Study the drawing (mm; zero at the part's minimum x, y, z) and answer. Coordinates: 2 decimals unless noted, no trailing zeros. Order: outer loops, then holes, each group sorted by start corner. A loop starts at its lowest first (then second) coordinate and runs counter-clockwise, first axis right, second up.
1. Flat-ended cylindrical pins translate along their axes: pin 1 Ø4.5 at (x, z) = (4.5, 2.5) entering from +Y; pin 2 Ø2.5 at (x, z) = (14.5, 2.5) entering from +Y. Find the tip coordinate at first contact, or state that the pin passes through.
2. The part is cut by section D-D, the plane x = 13.5. Give the vertices of the cut face in (y, z), then the cut area to 3 significant figures.
3. The part is cut by section C-C, the plane z = 17.5. Give the vertices of the cut face in (x, y), then the cut area to 3 significant figures.
4. The part is cut by section B-B, the plane x = 9.5. Give the vertices of the cut face in (y, z), then the cut area to 3 significant figures.
5. Determine the mould class of the marked faces 1, 2 and 3 for opening direction Z: +Z half, -Z half, draft (parallel to the pull), parting line (faces both ways), or undercut.
6. The part is cut by section A-A, the plane z = 10. Give the vertices of the cut face in (x, y), then the cut area to 3 significant figures.
7. Find the intervals of material crossed by probe 1 along X at (y, z) = (2.6, 2.5); probe 2 along Z at (x, y) = (4.25, 2.55); probe 3 along X at (y, z) = (3, 18.25), in increasing order.
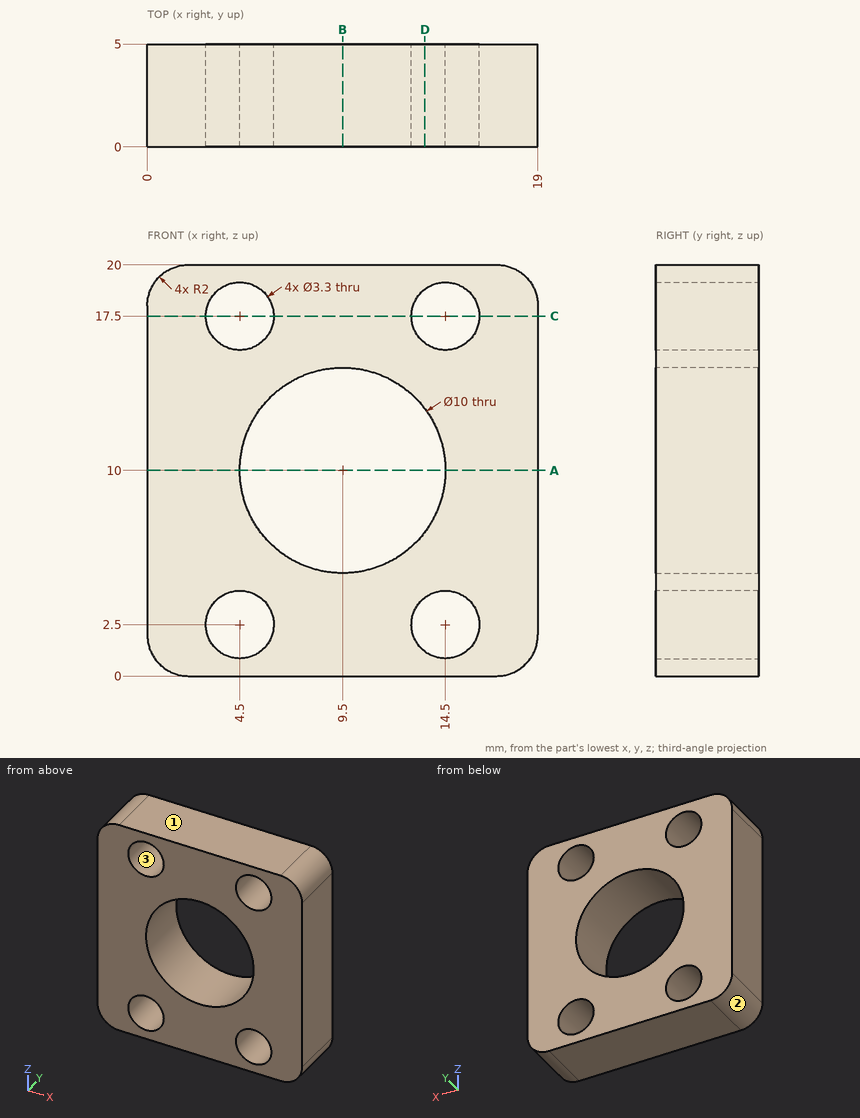
Geometry says:
1. pin 1: stops at y = 5
1. pin 2: passes through
2. outline: (0, 0) - (5, 0) - (5, 1.19) - (0, 1.19) - close; (0, 3.81) - (5, 3.81) - (5, 7) - (0, 7) - close; (0, 13) - (5, 13) - (5, 16.19) - (0, 16.19) - close; (0, 18.81) - (5, 18.81) - (5, 20) - (0, 20) - close
2. area: 43.8 mm2
3. outline: (0, 0) - (2.85, 0) - (2.85, 5) - (0, 5) - close; (6.15, 0) - (12.85, 0) - (12.85, 5) - (6.15, 5) - close; (16.15, 0) - (19, 0) - (19, 5) - (16.15, 5) - close
3. area: 62.0 mm2
4. outline: (0, 0) - (5, 0) - (5, 5) - (0, 5) - close; (0, 15) - (5, 15) - (5, 20) - (0, 20) - close
4. area: 50.0 mm2
5. face 1: +Z half
5. face 2: -Z half
5. face 3: undercut
6. outline: (0, 0) - (4.5, 0) - (4.5, 5) - (0, 5) - close; (14.5, 0) - (19, 0) - (19, 5) - (14.5, 5) - close
6. area: 45.0 mm2
7. probe 1: x = 0 to 2.85, 6.15 to 12.85, 16.15 to 19
7. probe 2: z = 0 to 0.87, 4.13 to 15.87, 19.13 to 20
7. probe 3: x = 0.02 to 3.03, 5.97 to 13.03, 15.97 to 18.98
